Geometry: see drawing. Coordinates: mm, zero at the bounding-box minimum. A direction names the side the tool comes from. Round coordinates to 2 decimals unless told otherwise and drop trailing zeros. Loops run counter-clockwise (first coordinate to the right, second up) from the corner with the lowest first, then second, coordinate; pieces in that order, holes last. Notation, with made-up numbers: (20.5, 3) - (30.5, 3) arc R15 ccw to (30.5, 20) - close; hole circle Ø5 at (-32.75, -14). An arc over 180 degrees is marked (long way). Use CSV: the item, a comma, the result in double quotes.
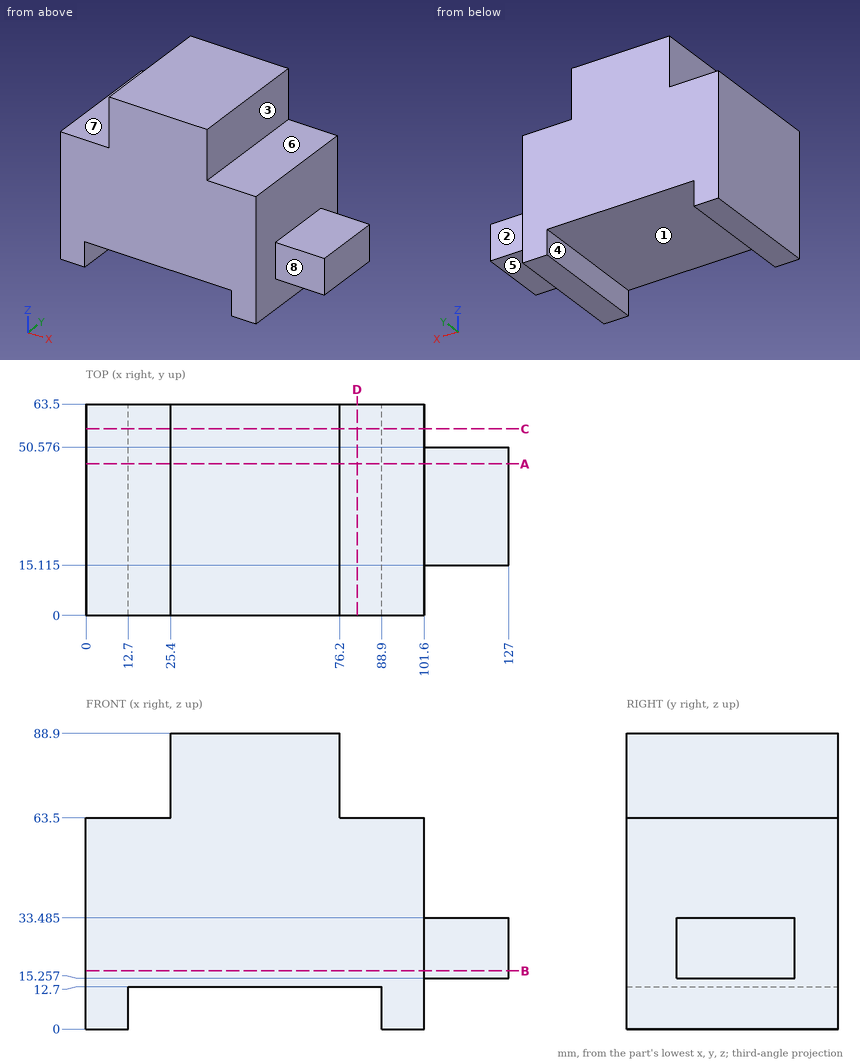
Item 1: Section B-B on z = 17.5. Return the cut outline in (x, y) (1 decimal).
Final values:
outline,"(0, 0) - (101.6, 0) - (101.6, 15.1) - (127, 15.1) - (127, 50.6) - (101.6, 50.6) - (101.6, 63.5) - (0, 63.5) - close"
Item 2: Material intervals for line 1 (X direction, y = 57, z = 67); line 2 (X direction, y = 31.5, z = 44); line 3 (Z direction, x = 44, y = 43), sorted ascending.
Final values:
line 1,"x = 25.4 to 76.2"
line 2,"x = 0 to 101.6"
line 3,"z = 12.7 to 88.9"
Item 3: Pin query (flat end, axial travel): P1, Ø20.5, axis at x = 117.5, y = 41.5, coming from the +Z side (1 decimal); P2, Ø20.5, axis at x = 112.5, y = 40.5, coming from the -Z side; P3, Ø20.5, axis at y = 17, z = 79.5, coming from the +X side. Return the tip coordinate at first contact, or that it passes through.
Final values:
P1,"stops at z = 33.5"
P2,"stops at z = 15.26"
P3,"stops at x = 76.2"
Item 4: Section A-A on y = 45.5. Return the cut outline in (x, z) (1 decimal).
Final values:
outline,"(0, 0) - (12.7, 0) - (12.7, 12.7) - (88.9, 12.7) - (88.9, 0) - (101.6, 0) - (101.6, 15.3) - (127, 15.3) - (127, 33.5) - (101.6, 33.5) - (101.6, 63.5) - (76.2, 63.5) - (76.2, 88.9) - (25.4, 88.9) - (25.4, 63.5) - (0, 63.5) - close"
Item 5: Section C-C on y = 56. Return the cut outline in (x, z), plus the area to 3 significant figures.
Final values:
outline,"(0, 0) - (12.7, 0) - (12.7, 12.7) - (88.9, 12.7) - (88.9, 0) - (101.6, 0) - (101.6, 63.5) - (76.2, 63.5) - (76.2, 88.9) - (25.4, 88.9) - (25.4, 63.5) - (0, 63.5) - close"
area,"6,770 mm²"
Item 6: Reachability of the marked faces 5, 6, 7 and 8 from +Z, -Z, +X, -X, +Y, -Y: full face, straight path, thin tool, end or side. Return the list, or none.
Final values:
face 5,"-Z, +X, +Y, -Y"
face 6,"+Z, +X, +Y, -Y"
face 7,"+Z, -X, +Y, -Y"
face 8,"+Z, -Z, +X, -Y"
Item 7: Section D-D on x = 81.5. Return the cut outline in (y, z), plus the area to 3 significant figures.
Final values:
outline,"(0, 12.7) - (63.5, 12.7) - (63.5, 63.5) - (0, 63.5) - close"
area,"3,230 mm²"
Item 8: Mould query, pull axis X, two halves, no side actions, for the marked faces 1, 2, 3 and 4. Classes: released by +X, released by -X, zero draft, split by the parting line, or undercut.
Final values:
face 1,"undercut"
face 2,"zero draft"
face 3,"released by +X"
face 4,"undercut"
